Check sheet for the drawn part. Datum: minimum x, y, z corner. Units: mm. Give positions to 0.01 mm unless a question says otherwise; leave off trailing zeros. Write each loop counter-clockwise with the first axis right and the second up, starting at its lowest first coordinate (ties: lowest second). Pieces come first, ordered by that corner, then holes. Notation, with made-up numbers: (73.5, 31) -> (94.5, 31) arc R19 cw to (94.5, 36) -> close; hole circle Ø4 at (77, -37.5). An arc over 180 degrees is marked (long way). Answer as CSV lines item,"result". Start each with the question number.
1) Material ranges on L1, parallel to X at y = 62, z = 60.5; L2, parallel to Z at x = 91.5, y = 49; L3, parallel to Z at x = 77, y = 26.5, recorded low to high.
2) Sectioned sample at A-A on y = 23.5. Record the cut outline in (x, z).
3) Gauge pin test, flat ends, axial feed: pin 1 Ø5 at (y, z) = (60.5, 45) entering from +X; pin 2 Ø10 at (y, z) = (12, 58) entering from -X; pin 3 Ø1 at (y, z) = (51, 39) entering from +X. Record the tip position at first contact, or that the pin passes through.
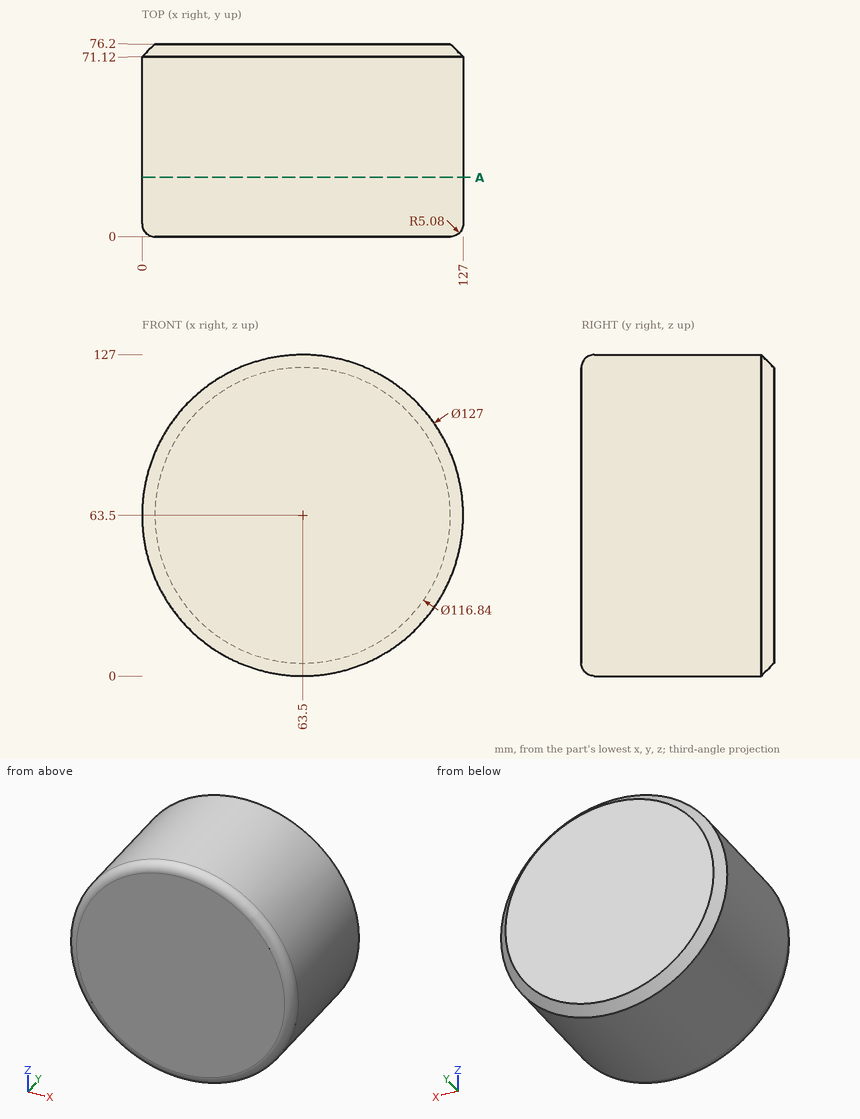
Ans:
1,L1,"x = 0.07 to 126.93"
1,L2,"z = 6.51 to 120.49"
1,L3,"z = 1.45 to 125.55"
2,outline,"circle Ø127 at (63.5, 63.5)"
3,pin 1,"stops at x = 124.95"
3,pin 2,"stops at x = 0"
3,pin 3,"stops at x = 122.29"
